Autodesk Inventor part; units mm, degrees
ref_plane "YZ Plane" through (0, 0, 0) normal (1, 0, 0) x (0, 1, 0)
ref_plane "XZ Plane" through (0, 0, 0) normal (0, 1, 0) x (-1, 0, 0)
ref_plane "XY Plane" through (0, 0, 0) normal (0, 0, 1) x (1, 0, 0)
sketch "Sketch1" plane through (0, 0, 0) normal (0, 1, 0) x (-1, 0, 0)
  line L0 (28.2, 28.2) -> (-28.2, 28.2)
  line L1 (-28.2, 28.2) -> (-28.2, -28.2)
  line L2 (-28.2, -28.2) -> (28.2, -28.2)
  line L3 (28.2, -28.2) -> (28.2, 28.2)
  line L4 (28.2, 28.2) -> (-28.2, -28.2) construction
  line L5 (-28.2, 28.2) -> (28.2, -28.2) construction
  line L6 (0, 28.2) -> (0, -28.2) construction
  line L7 (28.2, 0) -> (-28.2, 0) construction
  circle A0 centre (23.57, 23.57) radius 2.3
  circle A1 centre (23.57, -23.57) radius 2.3
  circle A2 centre (-23.57, 23.57) radius 2.3
  circle A3 centre (-23.57, -23.57) radius 2.3
  point P0 (0, 0)
  dimension "d0" = 56.4
  dimension "d1" = 56.4
  dimension "d2" = 4.6
  dimension "d5" = 47.14
  dimension "d6" = 47.14
extrude "Extrusion1" add sketch "Sketch1" along normal blind 10
sketch "Sketch2" plane through (0, 0, 0) normal (0, -1, 0) x (1, 0, 0)
  circle A0 centre (0, 0) radius 25.5
  dimension "d9" = 51
extrude "Extrusion2" add sketch "Sketch2" along normal blind 41
sketch "Sketch3" plane through (0, 10, 0) normal (0, 1, 0) x (1, 0, 0)
  circle A0 centre (0, 0) radius 19.05
  dimension "d12" = 38.1
extrude "Extrusion3" add sketch "Sketch3" along normal blind 1.6
sketch "Sketch4" plane through (0, 11.6, 0) normal (0, 1, 0) x (1, 0, 0)
  circle A0 centre (0, 0) radius 3.175
  dimension "d15" = 6.35
extrude "Extrusion4" add sketch "Sketch4" along normal blind 19
properties part number "Motor model"
Could you check a few things on this model? Use its own coordinates, in mm. A direction names the side the tool comes from. Give positions to 0.01 mm unless a question says otherwise; leave off trailing zeros. Order: outer loops, then holes, each group sorted by start corner. A loop starts at its lowest first (then second) coordinate and runs counter-clockwise, first axis right, second up. Notation, with made-up numbers: (20.5, 5.5) -> (66.5, 5.5) arc R12 cw to (66.5, 24.5) -> close; hole circle Ø11 at (55, -13.5). An arc over 180 degrees is marked (long way). Answer in a Markdown table with one row per item. Add a question column.
Item 1: We'd pull the mould along X, two halves only. Please class faces 4 (the cylindrical face through (-15.12, 10.79, -11.59)), 5 (the flat face through (0, 5, -28.2)), 6 (the cylindrical face through (-25.764, 4.93, 22.879)): pulls with the +X half, pulls with the -X half, needs draft (parallel to the pull), parting line crosses it, or undercut.
Item 2: Imagine slicing it at A-A (z = 23.57). List the corners of the cut face in (x, y) for me, and give its area (3 significant figures).
Item 3: Imagine slicing it at D-D (x = 23.5). List the corners of the cut face in (y, z) for me.
Item 4: Imagine slicing it at C-C (z = 0). List the corners of the cut face in (x, y) for me (3 decimals).
Item 5: For faces 1 (the cylindrical face through (-5.5, -20.2, 24.9)), 2 (the flat face through (0.4, 10, 19.2)), 3 (the flat face through (0, -41, 0)), which set-ups out of +Z, -Z, +X, -X, +Y, -Y let a thin tool reach every point of the face, with its end or its side?
Item 6: Please list where these lines run through material, in increasing order: probe 1 along Z at (x, y) = (23.57, 7.5); probe 2 along Z at (x, y) = (-23, 6); probe 3 along Y at (x, z) = (-10.5, 20.5).
Item 7: Imagine slicing it at B-B (x = 0). List the corners of the cut face in (y, z) for me (3 decimals).
Item 8: I'm going to push flat-ended pins straight in: P1, Ø6, axis at x = -23.57, z = 23.57, coming from the +Y side; P2, Ø3.5, axis at x = 23.57, z = 23.57, coming from the -Y side; P3, Ø5, axis at x = -9, y = -12, coming from the -Z side; P4, Ø5, axis at y = -23.5, z = 9, coming from the +X side. Where does each tip first touch, or does it pass through?
Result:
| question | item | result |
|---|---|---|
| 1 | face 4 | parting line crosses it |
| 1 | face 5 | needs draft |
| 1 | face 6 | undercut |
| 2 | outline | (-28.2, 0) -> (-25.87, 0) -> (-25.87, 10) -> (-28.2, 10) -> close; (-21.27, 0) -> (-9.73, 0) -> (-9.73, -41) -> (9.73, -41) -> (9.73, 0) -> (21.27, 0) -> (21.27, 10) -> (-21.27, 10) -> close; (25.87, 0) -> (28.2, 0) -> (28.2, 10) -> (25.87, 10) -> close |
| 2 | area | 1,270 mm2 |
| 3 | outline | (-41, -9.9) -> (0, -9.9) -> (0, -21.27) -> (10, -21.27) -> (10, 21.27) -> (0, 21.27) -> (0, 9.9) -> (-41, 9.9) -> close; (0, -28.2) -> (10, -28.2) -> (10, -25.87) -> (0, -25.87) -> close; (0, 25.87) -> (10, 25.87) -> (10, 28.2) -> (0, 28.2) -> close |
| 4 | outline | (-28.2, 0) -> (-25.5, 0) -> (-25.5, -41) -> (25.5, -41) -> (25.5, 0) -> (28.2, 0) -> (28.2, 10) -> (19.05, 10) -> (19.05, 11.6) -> (3.175, 11.6) -> (3.175, 30.6) -> (-3.175, 30.6) -> (-3.175, 11.6) -> (-19.05, 11.6) -> (-19.05, 10) -> (-28.2, 10) -> close |
| 5 | face 1 | -Y |
| 5 | face 2 | +Y |
| 5 | face 3 | +Z, -Z, +X, -X, -Y |
| 6 | probe 1 | -28.2 to -25.87, -21.27 to 21.27, 25.87 to 28.2 |
| 6 | probe 2 | -28.2 to -25.8, -21.34 to 21.34, 25.8 to 28.2 |
| 6 | probe 3 | -41 to 10 |
| 7 | outline | (-41, -25.5) -> (0, -25.5) -> (0, -28.2) -> (10, -28.2) -> (10, -19.05) -> (11.6, -19.05) -> (11.6, -3.175) -> (30.6, -3.175) -> (30.6, 3.175) -> (11.6, 3.175) -> (11.6, 19.05) -> (10, 19.05) -> (10, 28.2) -> (0, 28.2) -> (0, 25.5) -> (-41, 25.5) -> close |
| 8 | P1 | y = 10 |
| 8 | P2 | through |
| 8 | P3 | z = -24.66 |
| 8 | P4 | x = 24.66 |
